For this review, take the finished solid that the model builds, in its own axes (mm). A direction names the side the tool comes from. Round coordinates to 2 decimals unless told otherwise and drop trailing zeros. Loops run counter-clockwise (first coordinate to the right, second up) from the corner with the lowest first, then second, coordinate; pieces in that order, holes last.
1) Take a section at A-A (y = 0). State the section outline as (x, z) points, then the cut area to 3 significant figures.
2) Wall thickness on L1, parallel to Y at x = 25, z = -2.2; L2, parallel to Y at x = 25, z = -6.5; L3, parallel to X at y = 0, z = -1.3: over which ranges is each line inside the solid? List them lowest first.
3) Mouldability with a two-part tool opening along X and no side actions: class faces 1 (the flat face through (14, 16, -9)), 2 (the cylindrical face through (43.426, 16.896, -4.563)), 3 (the cylindrical face through (29.76, -3.65, -7.03)) as pulls with the +X half, pulls with the -X half, needs draft (parallel to the pull), parting line crosses it, or undercut.
4) Insertion check: pin 1 (4 mm diameter, centred on y = -2.5, z = -3, fed in from +X) (3 decimals); pin 2 (4 mm diameter, centred on y = 3, z = -0.5, fed in from -X); pin 3 (1 mm diameter, centred on y = 17.5, z = -4.5, fed in from -X). Each pin has a flat end and moves straight along its axis. Give the tip position at first contact, or say it passes through.
5) Tool access review of faces 4 (the cylindrical face through (20, 12, -3)), 5 (the cylindrical face through (27.343, 17.847, -7.028)), 6 (the cylindrical face through (29.76, 3.65, 0.51)): name each direction out of +Z, -Z, +X, -X, +Y, -Y from which nothing blocks a thin tool from reaching the whole face with its end or side.
6) Take a section at B-B (x = 25). State the section outline as (y, z) points, then the cut area to 3 significant figures.
7) Take a section at D-D (x = 41). State the section outline as (y, z) points.
8) Take a section at C-C (z = -7.25). State the section outline as (x, y) points, then the cut area to 3 significant figures.
Autodesk Inventor part; units mm, degrees
ref_plane "YZ Plane" through (0, 0, 0) normal (1, 0, 0) x (0, 1, 0)
ref_plane "XZ Plane" through (0, 0, 0) normal (0, 1, 0) x (-1, 0, 0)
ref_plane "XY Plane" through (0, 0, 0) normal (0, 0, 1) x (1, 0, 0)
sketch "Skizze4" plane through (0, 0, 0) normal (0, 1, 0) x (1, 0, 0)
  line L0 (25, 9) -> (25, -1)
  line L1 (25, 9) -> (7, 9)
  line L2 (12.1242, 0) -> (0, 0)
  line L3 (0, 0) -> (0, 9)
  line L4 (0, 9) -> (7, 9)
  line L5 (9.9688, 0) -> (19, 0)
  line L6 (19, 0) -> (19, -1)
  line L7 (19, -1) -> (25, -1)
  point P0 (6.0621, 0)
  dimension "d6" = 50
  dimension "d7" = 1
  dimension "d8" = 10
  dimension "d11" = 12
revolve "Umdrehung1" add sketch "Skizze4" angle 360 about axis through (25, 0, -9) along (0, 0, 1)
sketch "Skizze5" plane through (25, 0, -9) normal (0, 0, -1) x (-1, 0, 0)
  circle A0 centre (0, 0) radius 6
  circle A1 centre (0, 0) radius 18
  point P0 (25, 0)
  dimension "d20" = 36
extrude "Extrusion3" cut sketch "Skizze5" against normal blind 4
sketch "Skizze6" plane through (25, 0, -9) normal (0, 0, -1) x (-1, 0, 0)
  circle A0 centre (0, 0) radius 6
  point P0 (25, 0)
hole "Bohrung1" at (25, 0, -9) direction (0, 0, 1) diameter 8 end through all
sketch "Skizze7" plane through (25, 0, 0) normal (0, 0, 1) x (-1, 0, 0)
  circle A0 centre (0, 0) radius 4
  circle A1 centre (0, 0) radius 4
  line L0 (0, 0) -> (0, -45.1708) construction
  point P0 (25, 0)
  point P1 (12, 0)
  point P2 (-12, 0)
  dimension "d42" = 24
hole "Bohrung2" at (13, 0, 0) at (37, 0, 0) direction (0, 0, -1) diameter 10 end through all
pattern_circular "Runde Anordnung1" count 4 over 360 about axis through (25, 0, -4.5) along (0, 0, 1) of "Bohrung2"
properties part number "Schwungscheibe" material "Stahl, galvanisiert"
Response:
1. outline: (0, -9) - (7, -9) - (7, -5) - (8, -5) - (8, 0) - (0, 0) - close; (18, -5) - (19, -5) - (19, -9) - (21, -9) - (21, 1) - (19, 1) - (19, 0) - (18, 0) - close; (29, -9) - (31, -9) - (31, -5) - (32, -5) - (32, 0) - (31, 0) - (31, 1) - (29, 1) - close; (42, -5) - (43, -5) - (43, -9) - (50, -9) - (50, 0) - (42, 0) - close
1. area: 186 mm2
2. L1: y = -25 to -17, -7 to -4, 4 to 7, 17 to 25
2. L2: y = -25 to -18, -6 to -4, 4 to 6, 18 to 25
2. L3: x = 0 to 8, 18 to 21, 29 to 32, 42 to 50
3. face 1: needs draft
3. face 2: parting line crosses it
3. face 3: undercut
4. pin 1: stops at x = 49.995
4. pin 2: stops at x = 0.02
4. pin 3: stops at x = 6.67
5. face 4: +Z, -Z
5. face 5: -Z
5. face 6: +Z
6. outline: (-25, -9) - (-18, -9) - (-18, -5) - (-17, -5) - (-17, 0) - (-25, 0) - close; (-7, -5) - (-6, -5) - (-6, -9) - (-4, -9) - (-4, 1) - (-6, 1) - (-6, 0) - (-7, 0) - close; (4, -9) - (6, -9) - (6, -5) - (7, -5) - (7, 0) - (6, 0) - (6, 1) - (4, 1) - close; (17, -5) - (18, -5) - (18, -9) - (25, -9) - (25, 0) - (17, 0) - close
6. area: 186 mm2
7. outline: (-19.21, -9) - (-8.25, -9) - (-8.25, -5) - (-3, -5) - (-3, 0) - (-19.21, 0) - close; (3, -5) - (8.25, -5) - (8.25, -9) - (19.21, -9) - (19.21, 0) - (3, 0) - close
8. outline: circle Ø50 at (25, 0); circle Ø12 at (25, 0); hole circle Ø36 at (25, 0); hole circle Ø8 at (25, 0)
8. area: 1,010 mm2
